Check sheet for the drawn part. Datum: minimum x, y, z corner. Units: mm. A direction names the side the tool comes from. Give positions to 0.01 mm unless a question says otherwise; leave off trailing zeros. Write each loop counter-clockwise with the first axis right and the second up, starting at its lowest first coordinate (ties: lowest second). Pieces come first, ordered by that corner, then holes. Notation, with made-up numbers: (-6, -19) - (25, -19) arc R23 cw to (25, 16) - close; hole circle Ø7 at (67.25, 44.5). An arc over 180 degrees is marked (long way). Answer as a JSON object with one key per item and string values. Group by question number.
Item 1: Draft check along X on the marked faces 4, 5 and 6. Enter one of: +X half, -X half, draft (parallel to the pull), parting line (faces both ways), or undercut.
Item 2: Tool access check on the marked faces 1, 2 and 3. Record the directions out of +Z, -Z, +X, -X, +Y, -Y that give a thin tool (end or side, any length) a straight path to the whole face; none if there is none.
Item 3: Sectioned sample at B-B, the plane z = 5.25. Record the boundary of the cut face in (x, y).
Item 4: Sectioned sample at D-D, the plane y = 10.25. Record the boundary of the cut face in (x, z) (3 decimals).
Item 5: Scan lines: line 1 along Y through (x, z) = (2.5, 10.25); line 2 along X through (y, z) = (13.25, 10.5); line 3 along Y through (x, z) = (9, 11.25). Record each from-to range of solid material in increasing order. Write a range as [from, to].
Item 6: Go/stop test with flat-tipped pins: pin 1 (8 mm diameter, centred on x = 7, y = 12.5, fed in from -Z) (3 decimals); pin 2 (0.6 mm diameter, centred on y = 13, z = 11, fed in from -X); pin 3 (5 mm diameter, centred on x = 6.875, z = 6.875, fed in from +Y); pin 4 (3 mm diameter, centred on y = 7, z = 3.5, fed in from -X). Record where each tip stops, or that it passes through.
Item 7: Sectioned sample at A-A, the plane y = 12.75. Record the boundary of the cut face in (x, z) (3 decimals).
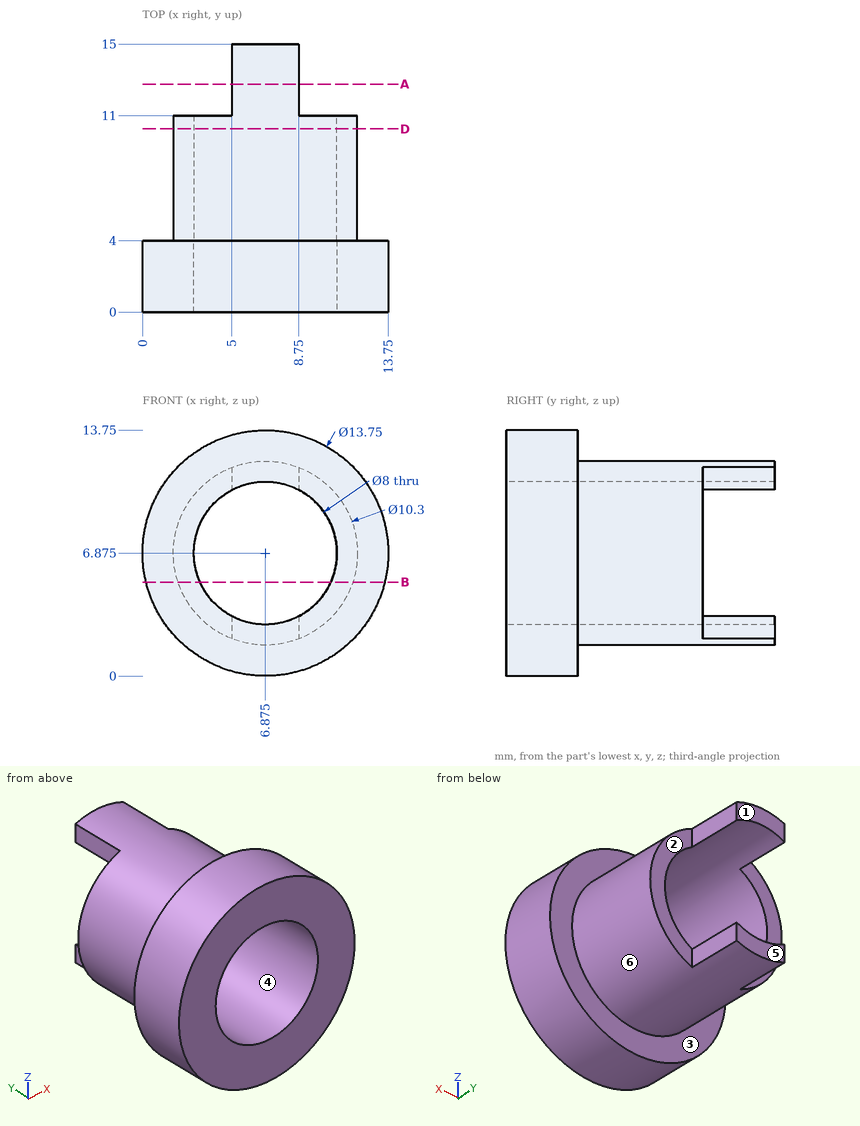
Geometry check:
{
 "1": {"face 4": "undercut", "face 5": "draft", "face 6": "parting line"},
 "2": {"face 1": "+Z, -Z, +X, -X, +Y", "face 2": "+Z, -Z, +X, +Y", "face 3": "+Y"},
 "3": {"outline": "(0.19, 0) - (3.22, 0) - (3.22, 11) - (1.99, 11) - (1.99, 4) - (0.19, 4) - close; (10.53, 0) - (13.56, 0) - (13.56, 4) - (11.76, 4) - (11.76, 11) - (10.53, 11) - close"},
 "4": {"outline": "circle Ø10.3 at (6.875, 6.875); hole circle Ø8 at (6.875, 6.875)"},
 "5": {"line 1": "[0, 4]", "line 2": "[5, 5.18], [8.57, 8.75]", "line 3": "[0, 11]"},
 "6": {"pin 1": "z = 1.725", "pin 2": "x = 5", "pin 3": "through", "pin 4": "x = 2.08"},
 "7": {"outline": "(5, 2.078) arc R5.15 ccw to (8.75, 2.078) - (8.75, 3.342) arc R4 cw to (5, 3.342) - close; (5, 10.408) arc R4 cw to (8.75, 10.408) - (8.75, 11.672) arc R5.15 ccw to (5, 11.672) - close"}
}
